The drawing under review shows one solid part. Ordinate dimensions are in mm from its lowest x, y, z. Coordinates: 2 decimals unless noted, no trailing zeros. Order: outer loops, then holes, each group sorted by start corner. A loop starts at its lowest first (then second) coordinate and runs counter-clockwise, first axis right, second up.
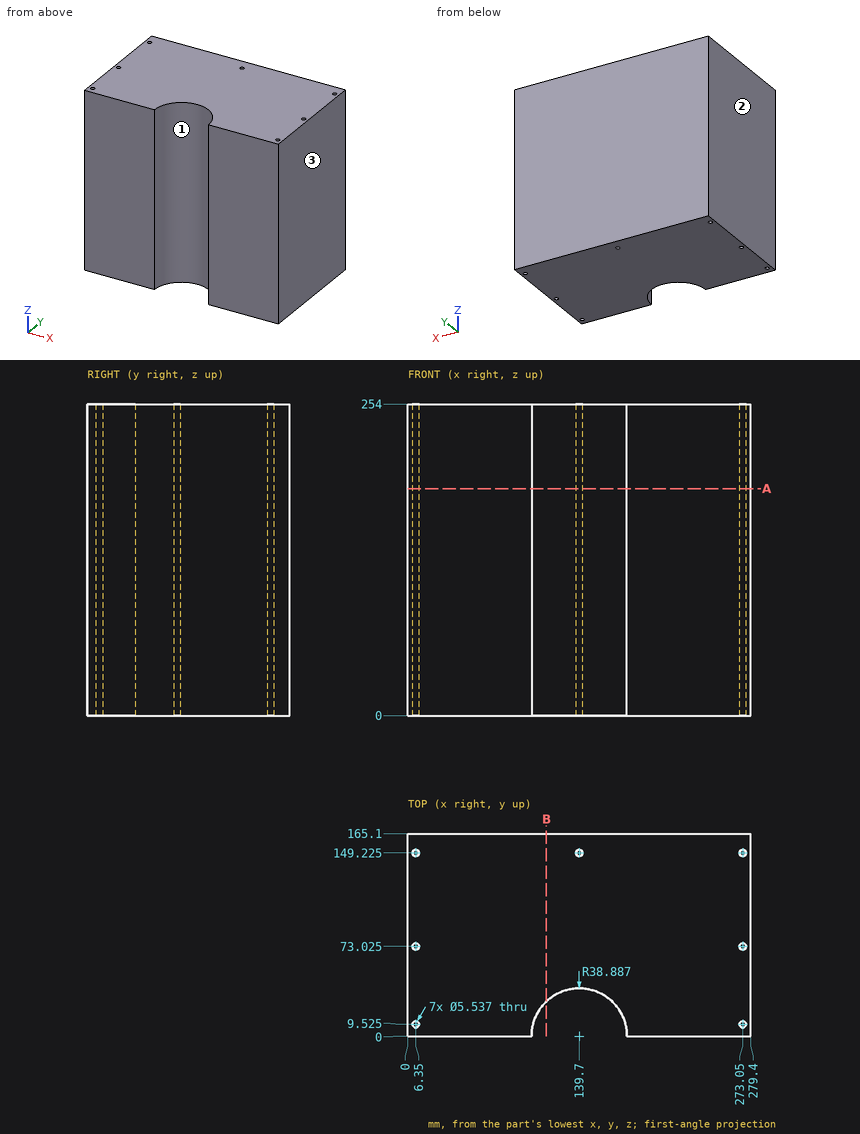
1. Add section B-B (x = 113). Give the boundary of the cut face in (y, z).
2. To check wall thickness, follow line 1 (Y direction, x = 273, z = 160); line 2 (X direction, y = 11, z = 74); line 3 (X direction, y = 30, z = 13) (1 decimal). State the ranges of each line that lie inside material, in increasing order.
3. Add section A-A (z = 185). State how many separate pieces and enclosed holes the cut face has, and give its area (3 significant figures).
4. Insertion check: pin 1 (5 mm diameter, centred on y = 110, z = 107, fed in from -X); pin 2 (5 mm diameter, centred on x = 171.5, z = 125.5, fed in from -Y) (1 decimal); pin 3 (2 mm diameter, centred on x = 126, z = 175, fed in from -Y). Each pin has a flat end and moves straight along its axis. Give the tip position at first contact, or say it passes through.
5. Mouldability with a two-part tool opening along X and no side actions: class the marked faces 1, 2 and 3 as pulls with the +X half, pulls with the -X half, needs draft (parallel to the pull), parting line crosses it, or undercut.
Solution:
1. outline: (28.27, 0) - (165.1, 0) - (165.1, 254) - (28.27, 254) - close
2. line 1: y = 0 to 6.76, 12.29 to 70.26, 75.79 to 146.46, 151.99 to 165.1
2. line 2: x = 0 to 4.01, 8.69 to 102.4, 177 to 270.71, 275.39 to 279.4
2. line 3: x = 0 to 115, 164.4 to 279.4
3. separate pieces: 1
3. enclosed holes: 7
3. area: 43,600 mm2
4. pin 1: stops at x = 0
4. pin 2: stops at y = 18.3
4. pin 3: stops at y = 36
5. face 1: undercut
5. face 2: pulls with the -X half
5. face 3: pulls with the +X half
